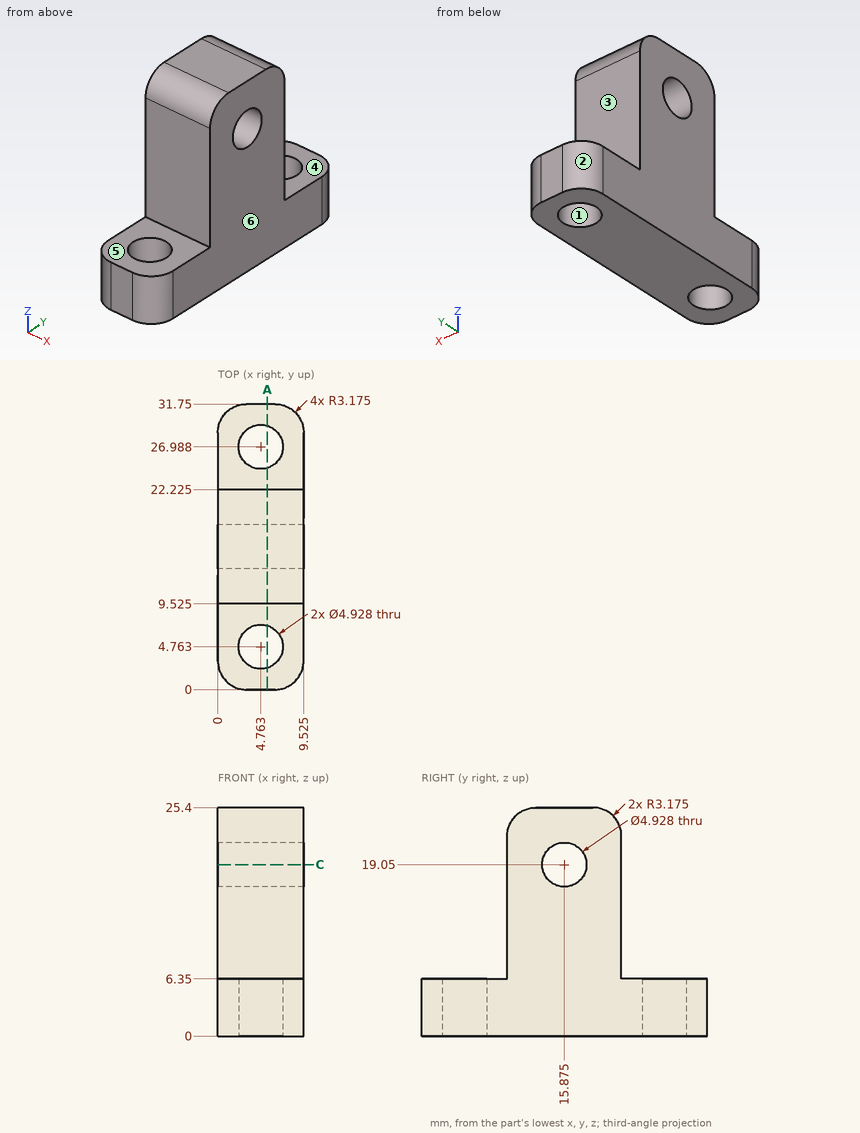
Study the drawing (mm; zero at the part's minimum x, y, z) and answer. A direction names the side the tool comes from. Coordinates: 2 decimals unless noted, no trailing zeros. Loops run counter-clockwise (first coordinate to the right, second up) from the corner with the lowest first, then second, coordinate; pieces in that order, holes last. Notation, with made-up numbers: (11.25, 6) -> (50.25, 6) arc R17 cw to (50.25, 20) -> close; hole circle Ø6 at (52, 10). An arc over 180 degrees is marked (long way). Write each question's results on one line, items separated by ' | '. Start each with the question number.
1) Consider line 1 along Y through (x, z) = (7, 4.75) (1 decimal); line 2 along Y through (x, z) = (6.5, 19.05) (1 decimal); line 3 along Y through (x, z) = (5.25, 13.5) (1 decimal). Determine where each line is inside the solid, lowest interval first.
2) Flat-ended cylindrical pins translate along their axes: P1, Ø5, axis at x = 4.5, y = 28.5, coming from the +Z side; P2, Ø3, axis at x = 6.5, z = 13, coming from the +Y side (1 decimal). Find the tip coordinate at first contact, or state that the pin passes through.
3) For the marked faces 4, 5 and 6, determine the directions among +Z, -Z, +X, -X, +Y, -Y from which every point of the face is accessible in a straight line to the end or side of a thin tool.
4) Find section C-C on z = 19.05. Determine the outline of the cut face in (x, y) (1 decimal).
5) Find section A-A on x = 5.5. Count the separate pieces of the cut face and the enclosed holes in it.
6) The mould has two halves that part along X. Classify the marked faces 1, 2 and 3: pulls with the +X half, pulls with the -X half, needs draft (parallel to the pull), parting line crosses it, or undercut.
Response values:
1) line 1: y = 0.1 to 3.7, 5.8 to 26, 28 to 31.7 | line 2: y = 9.5 to 13.4, 18.3 to 22.2 | line 3: y = 9.5 to 22.2
2) P1: stops at z = 6.35 | P2: stops at y = 22.2
3) face 4: +Z, +X, -X, +Y | face 5: +Z, +X, -X, -Y | face 6: +Z, -Z, +X, +Y, -Y
4) outline: (0, 9.5) -> (9.5, 9.5) -> (9.5, 13.4) -> (0, 13.4) -> close; (0, 18.3) -> (9.5, 18.3) -> (9.5, 22.2) -> (0, 22.2) -> close
5) separate pieces: 3 | enclosed holes: 1
6) face 1: undercut | face 2: pulls with the -X half | face 3: needs draft
